Model file for the job. Use its own axes, mm. Give positions to 0.01 mm unless a question says otherwise; leave off trailing zeros. Use CSV: the item, a comma, the result in double quotes. Start each with the question number.
(1) Probe L1, parallel to Y at x = -25.5, z = 13.5 (3 decimals); L2, parallel to X at y = 4.5, z = -10; L3, parallel to X at y = -5.75, z = -9 (3 decimals). List the from-to ranges inside material, lowest first.
(2) Pull direction X, two halves, no side cores. Call faces 1 (the flat face through (-16, -9.525, 0)), 2 (the flat face through (-9.525, -5, 0)): +X half, -X half, draft (parallel to the pull), parting line (faces both ways), or undercut.
(3) Drop flat-ended pins along their axis: pin 1 Ø1.5 at (x, y) = (-6, 6) entering from +Z; pin 2 Ø1 at (x, z) = (-29.5, -25) entering from -Y; pin 3 Ø8 at (x, y) = (-22, 0) entering from -Z. Give the stop position or say it passes through.
Autodesk Inventor part; units mm, degrees
ref_plane "YZ Plane" through (0, 0, 0) normal (1, 0, 0) x (0, 1, 0)
ref_plane "XZ Plane" through (0, 0, 0) normal (0, 1, 0) x (-1, 0, 0)
ref_plane "XY Plane" through (0, 0, 0) normal (0, 0, 1) x (1, 0, 0)
sketch "Sketch1" plane through (0, 0, 0) normal (0, 1, 0) x (-1, 0, 0)
  ellipse E0 centre (0, 0) end of major axis (0, -40.64) minor radius 50.8 (0, -40.64) -> (0, 40.64) ccw
  line L0 (0, 40.64) -> (0, -40.64)
  ellipse E1 centre (0, 0) end of major axis (0, -31.75) minor radius 25.4 (0, -31.75) -> (0, 31.75) ccw
  line L1 (0, 40.64) -> (0, -40.64)
  point P0 (0, -31.75)
  point P1 (0, 31.75)
  dimension "d0" = 50.8
  dimension "d1" = 40.64
  dimension "d2" = 25.4
  dimension "d3" = 31.75
extrude "Extrusion1" add sketch "Sketch1" along normal blind 9.525
extrude "Extrusion2" add sketch "Sketch1" against normal blind 9.525 contours L0 E1
sketch "Sketch3" plane through (0, -9.525, 0) normal (0, -1, 0) x (1, 0, 0)
  line L0 (0, -31.75) -> (0, 31.75)
  ellipse E0 centre (0, 0) end of major axis (0, -31.75) minor radius 25.4 (0, 31.75) -> (0, -31.75) ccw
  line L1 (0, 40.64) -> (0, -40.64)
  ellipse E1 centre (0, 0) end of major axis (0, -31.75) minor radius 25.4 (0, 31.75) -> (0, -31.75) ccw
  line L2 (-9.525, 29.433) -> (-9.525, -29.433)
  ellipse E2 centre (0, 0) end of major axis (0, -31.75) minor radius 25.4 (0, 31.75) -> (-9.525, 29.433) ccw
  ellipse E3 centre (0, 0) end of major axis (0, -31.75) minor radius 25.4 (-9.525, -29.433) -> (0, -31.75) ccw
  point P0 (-9.525, -29.433)
  dimension "d8" = 9.525
extrude "Extrusion3" cut sketch "Sketch3" against normal blind 9.525 contours E0 L2 L0
properties part number "pryBarHolder"
Answer block:
1,L1,"y = 0 to 9.525"
1,L2,"x = -49.24 to 0"
1,L3,"x = -24.358 to -9.525"
2,face 1,"draft"
2,face 2,"+X half"
3,pin 1,"stops at z = 40.42"
3,pin 2,"stops at y = 0"
3,pin 3,"stops at z = -38"
